from build123d import *

# Parameters (mm, degrees)
SKETCH_1_W               = 40
SKETCH_1_H               = 44
SKETCH_1_R               = 4.5
EXTRUDE_1_DEPTH          = 5
SKETCH_2_R               = 5.25
CUT_EXTRUDE_1_DEPTH      = 1
CUT_EXTRUDE_2_REACH      = 7
SKETCH_3_W               = 19
SKETCH_3_H               = 20.351449313
SKETCH_4_W               = 40
SKETCH_4_H               = 5
EXTRUDE_2_DEPTH          = 6
EXTRUDE_3_DEPTH          = 4
SKETCH_6_R               = 1.5
CUT_EXTRUDE_4_DEPTH      = 5
CUT_EXTRUDE_5_DEPTH      = 0.5
CUT_EXTRUDE_5_DEPTH_BACK = 2.5
EXTRUDE_4_DEPTH          = 3
EXTRUDE_5_DEPTH          = 3


with BuildPart() as part:
    # 草图1 → 凸台-拉伸1 (new body)
    with BuildSketch(Plane(origin=(0, 0, 0), x_dir=(0, 0, -1), z_dir=(1, 0, 0))):
        with Locations((9, -5)):
            Rectangle(SKETCH_1_W, SKETCH_1_H)
        Circle(SKETCH_1_R, mode=Mode.SUBTRACT)
        with Locations((18, 6)):
            Circle(SKETCH_1_R, mode=Mode.SUBTRACT)
        with Locations((11.543885882, -13.351449313)):
            Circle(SKETCH_1_R, mode=Mode.SUBTRACT)
    extrude(amount=EXTRUDE_1_DEPTH)

    # 草图2 → 切除-拉伸1 (cut)
    with BuildSketch(Plane.ZY.offset(-5)):
        with Locations((-18, 6)):
            Circle(SKETCH_2_R)
        Circle(SKETCH_2_R)
        with Locations((-11.543885882, -13.351449313)):
            Circle(SKETCH_2_R)
    extrude(amount=CUT_EXTRUDE_1_DEPTH, mode=Mode.SUBTRACT)

    # 草图3 → 切除-拉伸2 (cut, up to next)
    with BuildSketch(Plane(origin=(5, 0, 0), x_dir=(0, 0, -1), z_dir=(1, 0, 0)), mode=Mode.PRIVATE) as cut_extrude_2_sk1:
        with Locations((19.5, 6.824275344)):
            Rectangle(SKETCH_3_W, SKETCH_3_H)
    cut_extrude_2_tool1 = extrude(cut_extrude_2_sk1.sketch, amount=-CUT_EXTRUDE_2_REACH, mode=Mode.PRIVATE) & part.part
    add(cut_extrude_2_tool1.solids().sort_by_distance((5, 6.824275, -19.5))[0], mode=Mode.SUBTRACT)

    # 草图4 → 凸台-拉伸2 (add)
    with BuildSketch(Plane(origin=(5, 0, 0), x_dir=(0, 0, -1), z_dir=(1, 0, 0))):
        with Locations((9, -24.5)):
            Rectangle(SKETCH_4_W, SKETCH_4_H)
    extrude(amount=EXTRUDE_2_DEPTH)

    # 草图5 → 凸台-拉伸3 (add)
    with BuildSketch(Plane.XZ.offset(27)):
        Polygon((0, 11), (11, 11), (11, 9), (8.8, 9), (5.5, 6), (2.2, 9), (0, 9), align=None)
        with BuildLine():
            Line((0, -29), (9, -29))
            ThreePointArc((9, -29), (11, -27), (9, -25))
            Line((9, -25), (0, -25))
            Line((0, -25), (0, -29))
        make_face()
    extrude(amount=EXTRUDE_3_DEPTH)

    # 草图6 → 切除-拉伸4 (cut)
    with BuildSketch(Plane.XZ.offset(27)):
        with Locations((6.5, -19)):
            Circle(SKETCH_6_R)
        with Locations((6.5, 1)):
            Circle(SKETCH_6_R)
    extrude(amount=-CUT_EXTRUDE_4_DEPTH, mode=Mode.SUBTRACT)

    # 草图7 → 切除-拉伸5 (cut, two sides)
    with BuildSketch(Plane(origin=(0, -22, 0), x_dir=(-1, 0, 0), z_dir=(0, 1, 0))) as cut_extrude_5_sk:
        Polygon((-9.704293994, -19), (-8.102146997, -21.775), (-4.897853003, -21.775), (-3.295706006, -19), (-4.897853003, -16.225), (-8.102146997, -16.225), align=None)
        Polygon((-9.704293994, 1), (-8.102146997, -1.775), (-4.897853003, -1.775), (-3.295706006, 1), (-4.897853003, 3.775), (-8.102146997, 3.775), align=None)
    extrude(amount=CUT_EXTRUDE_5_DEPTH, mode=Mode.SUBTRACT)
    extrude(cut_extrude_5_sk.sketch, amount=-CUT_EXTRUDE_5_DEPTH_BACK, mode=Mode.SUBTRACT)

    # 草图8 → 凸台-拉伸4 (add)
    with BuildSketch(Plane.XY.offset(11)):
        Polygon((5, -22), (11, -22), (5, -5), align=None)
    extrude(amount=-EXTRUDE_4_DEPTH)

    # 草图9 → 凸台-拉伸5 (add)
    with BuildSketch(Plane(origin=(0, 0, -29), x_dir=(-1, 0, 0), z_dir=(0, 0, -1))):
        Polygon((-5, -22), (-11, -22), (-5, -5), align=None)
    extrude(amount=-EXTRUDE_5_DEPTH)


solid = part.part
Work out the finished part from the listing and answer in its coordinate system (mm). A direction names the side the tool comes from. Give positions to 0.01 mm unless a question says otherwise; leave off trailing zeros. Write each loop counter-clockwise with the first axis right and the second up, starting at its lowest first coordinate (ties: lowest second). Pieces come first, ordered by that corner, then holes.
Q1. For a pull along X with two mould halves and no side action, classify faces 1 (the face through (11, -24, -9)), 2 (the face through (5, -27, -9)), 3 (the face through (8.914, -23.232, -20.368)) as released by +X, released by -X, zero draft, split by the parting line, or undercut.
Answer:
face 1: released by +X
face 2: zero draft
face 3: undercut
Q2. The part is cut by section B-B on y = -26. Give the vertices of the cut face in (x, z), and give its area (3 significant figures).
Answer:
outline: (0, -29) - (11, -29) - (11, 11) - (0, 11) - close; hole circle Ø3 at (6.5, -19); hole circle Ø3 at (6.5, 1)
area: 426 mm2
Q3. The part is cut by section D-D on y = -16.5. Give the vertices of the cut face in (x, z).
Answer:
outline: (0, -29) - (9.06, -29) - (9.06, -26) - (5, -26) - (5, -15.74) - (4, -15.74) - (4, -14.76) - (0, -14.76) - close; (0, -8.33) - (4, -8.33) - (4, -7.34) - (5, -7.34) - (5, 8) - (9.06, 8) - (9.06, 11) - (0, 11) - close
Q4. The part is cut by section A-A on y = 0. Give the vertices of the cut face in (x, z).
Answer:
outline: (0, -10) - (5, -10) - (5, -5.25) - (4, -5.25) - (4, -4.5) - (0, -4.5) - close; (0, 4.5) - (4, 4.5) - (4, 5.25) - (5, 5.25) - (5, 11) - (0, 11) - close
Q5. The part is cut by section C-C on x = 6.5. Give the vertices of the cut face in (y, z) (3 decimals).
Answer:
outline: (-31, -29) - (-9.25, -29) - (-9.25, -26) - (-22, -26) - (-22, -21.775) - (-24.5, -21.775) - (-24.5, -20.5) - (-27, -20.5) - (-27, -25) - (-31, -25) - close; (-31, 6.909) - (-27, 6.909) - (-27, 2.5) - (-24.5, 2.5) - (-24.5, 3.775) - (-22, 3.775) - (-22, 8) - (-9.25, 8) - (-9.25, 11) - (-31, 11) - close; (-27, -17.5) - (-24.5, -17.5) - (-24.5, -16.225) - (-22, -16.225) - (-22, -1.775) - (-24.5, -1.775) - (-24.5, -0.5) - (-27, -0.5) - close
Q6. Straight lines are drawn through the part: L1, parallel to Z at x = 6.5, y = -25; L2, parallel to Y at x = 2, z = -11.5; L3, parallel to Z at x = 2.1, y = 0. For each, find the intervals that lie inside material, in ascending order.
Answer:
L1: z = -29 to -20.5, -17.5 to -0.5, 2.5 to 11
L2: y = -27 to -17.85, -8.85 to -3.35
L3: z = -10 to -4.5, 4.5 to 11
Q7. Given pin 1 (8 mm diameter, centred on y = -14.5, z = 5.5, fed in from +X) (3 decimals); pin 2 (6 mm diameter, centred on y = -14, z = 1.5, fed in from +X); pin 3 (0.5 mm diameter, centred on x = 4, z = -19, fed in from -Y), each flat-ended and moving along its own axis, determine where each tip first touches the part or whether it passes through.
Answer:
pin 1: stops at x = 9.455
pin 2: stops at x = 5
pin 3: stops at y = -27
Q8. A tool of negligible diameter and unlimited length cuts with its end or side. For faces 4 (the face through (3, -3.351, -19)), 5 (the face through (10.6, -27, -28.6)), 6 (the face through (4.5, 1.6, 5)), from which of +Z, -Z, +X, -X, +Y, -Y can it reach the whole face along a straight path? Write none if from no direction.
Answer:
face 4: -Z, +X, -X, +Y
face 5: -Z, +X, -Y
face 6: +X
